Geometry check sheet. Reference: the model listing, model coordinates, mm. A direction names the side the tool comes from. Coordinates: 2 decimals unless noted, no trailing zeros. Order: outer loops, then holes, each group sorted by start corner. A loop starts at its lowest first (then second) coordinate and runs counter-clockwise, first axis right, second up.
```python
from build123d import *

# Parameters (mm, degrees)
SKETCH1_W                                           = 50
SKETCH1_H                                           = 20
BOSS_EXTRUDE1_DEPTH                                 = 25
CBORE_FOR_M6_HEX_SOCKET_HEAD_CAP_SCREW1_D           = 6.4
CBORE_FOR_M6_HEX_SOCKET_HEAD_CAP_SCREW1_CBORE_D     = 11
CBORE_FOR_M6_HEX_SOCKET_HEAD_CAP_SCREW1_CBORE_DEPTH = 12
M5_CLEARANCE_HOLE1_D                                = 5.5
CUT_EXTRUDE1_DEPTH                                  = 4.5
FILLET1_R                                           = 1
CHAMFER1_SIZE                                       = 0.6


with BuildPart() as part:
    # Sketch1 → Boss-Extrude1 (new body)
    with BuildSketch(Plane.XY):
        Rectangle(SKETCH1_W, SKETCH1_H)
    extrude(amount=BOSS_EXTRUDE1_DEPTH)

    # CBORE for M6 Hex Socket Head Cap Screw1 (through all)
    with Locations(Plane.XY.offset(25)):
        with Locations((-12.5, 0), (12.5, 0)):
            CounterBoreHole(CBORE_FOR_M6_HEX_SOCKET_HEAD_CAP_SCREW1_D / 2, CBORE_FOR_M6_HEX_SOCKET_HEAD_CAP_SCREW1_CBORE_D / 2, CBORE_FOR_M6_HEX_SOCKET_HEAD_CAP_SCREW1_CBORE_DEPTH)

    # M5 Clearance Hole1 (through all)
    with Locations(Plane(origin=(0, -10, 0), x_dir=(-1, 0, 0), z_dir=(0, -1, 0))):
        with Locations((0, -15)):
            Hole(M5_CLEARANCE_HOLE1_D / 2)

    # Sketch7 → Cut-Extrude1 (cut)
    with BuildSketch(Plane(origin=(0, 10, 0), x_dir=(1, 0, 0), z_dir=(0, 1, 0))):
        Polygon((3.9, -12.74833395), (0, -10.4966679), (-3.9, -12.74833395), (-3.9, -17.25166605), (0, -19.5033321), (3.9, -17.25166605), align=None)
    extrude(amount=-CUT_EXTRUDE1_DEPTH, mode=Mode.SUBTRACT)

    # Fillet1
    fillet1_edges = [part.edges().sort_by_distance(p)[0] for p in [
        (-25, 10, 12.5),
        (25, 10, 12.5),
        (25, -10, 12.5),
        (-25, -10, 12.5),
    ]]
    fillet(fillet1_edges, radius=FILLET1_R)

    # Chamfer1
    chamfer1_edges = [part.edges().sort_by_distance(p)[0] for p in [
        (7, 0, 25),
        (15.7, 0, 0),
        (-18, 0, 25),
        (-9.3, 0, 0),
        (-25, 0, 0),
        (-25, 0, 25),
        (0, 10, 0),
        (25, 0, 0),
        (0, -10, 0),
        (24.707106781, -9.707106781, 0),
        (24.707106781, 9.707106781, 0),
        (-24.707106781, -9.707106781, 0),
        (-24.707106781, 9.707106781, 0),
        (0, 10, 25),
        (0, -10, 25),
        (25, 0, 25),
        (24.707106781, -9.707106781, 25),
        (24.707106781, 9.707106781, 25),
        (-24.707106781, -9.707106781, 25),
        (-24.707106781, 9.707106781, 25),
    ]]
    chamfer(chamfer1_edges, length=CHAMFER1_SIZE)


solid = part.part
```
Item 1: Thickness scan on line 1 along X through (y, z) = (2.25, 15); line 2 along Y through (x, z) = (-12.5, 18.5); line 3 along Y through (x, z) = (12.5, 8.5). Record the ranges inside material, lowest first.
Item 2: Sectioned sample at A-A (y = 0). Give the number of separate pieces and of enclosed holes in the cut face, and give its area (3 significant figures).
Item 3: Release check for a two-part mould opening along Z. For faces 1 (the face through (-1.98, 7.78, 18.36)), 2 (the face through (24.44, 9.45, 24.77)), 3 (the face through (0, 10, 10)), 4 (the face through (-0.358, -2.141, 12.273)) record: pulls with the +Z half, pulls with the -Z half, needs draft (parallel to the pull), parting line crosses it, or undercut.
Item 4: Tool access check on faces 5 (the face through (-25, 0, 12)), 6 (the face through (3.9, 8, 15)), 7 (the face through (14.9, -2.4, 13)). Record the directions out of +Z, -Z, +X, -X, +Y, -Y that give a thin tool (end or side, any length) a straight path to the whole face; none if there is none.
Item 5: Sectioned sample at D-D (y = -8.5). Record the cut outline in (x, z), and give its area (3 significant figures).
Item 6: Depth check by flat-ended pin: P1, Ø5.5, axis at x = 11.5, y = -2, coming from the +Z side; P2, Ø2.5, axis at x = 1, z = 13, coming from the +Y side. Enter the tip coordinate at first touch or a pass-through.
Item 7: Sectioned sample at B-B (z = 21.5). Record the cut outline in (x, y), and give its area (3 significant figures).
Item 8: Sectioned sample at C-C (x = 12.5). Record the cut outline in (y, z), and give its area (3 significant figures).
Geometry check:
1. line 1: x = -25 to -17.52, -7.48 to -2.75, 2.75 to 7.48, 17.52 to 25
1. line 2: y = -10 to -5.5, 5.5 to 10
1. line 3: y = -10 to -3.2, 3.2 to 10
2. separate pieces: 3
2. enclosed holes: 1
2. area: 794 mm2
3. face 1: undercut
3. face 2: pulls with the +Z half
3. face 3: needs draft
3. face 4: undercut
4. face 5: +Z, -Z, -X, +Y, -Y
4. face 6: +Y
4. face 7: +Z
5. outline: (-25, 0.6) - (-24.4, 0) - (24.4, 0) - (25, 0.6) - (25, 24.4) - (24.4, 25) - (-24.4, 25) - (-25, 24.4) - close; hole circle Ø5.5 at (0, 15)
5. area: 1,230 mm2
6. P1: stops at z = 13
6. P2: stops at y = 5.5
7. outline: (-25, -9) arc R1 ccw to (-24, -10) - (24, -10) arc R1 ccw to (25, -9) - (25, 9) arc R1 ccw to (24, 10) - (-24, 10) arc R1 ccw to (-25, 9) - close; hole circle Ø11 at (-12.5, 0); hole circle Ø11 at (12.5, 0)
7. area: 809 mm2
8. outline: (-10, 0.6) - (-9.4, 0) - (-3.8, 0) - (-3.2, 0.6) - (-3.2, 13) - (-5.5, 13) - (-5.5, 24.4) - (-6.1, 25) - (-9.4, 25) - (-10, 24.4) - close; (3.2, 0.6) - (3.8, 0) - (9.4, 0) - (10, 0.6) - (10, 24.4) - (9.4, 25) - (6.1, 25) - (5.5, 24.4) - (5.5, 13) - (3.2, 13) - close
8. area: 283 mm2
